```python
from build123d import *

# Parameters (mm, degrees)
F1_DEPTH = 3.175
F2_R     = 3.175
F3_DEPTH = 6.351


with BuildPart() as f1:
    # F0 (on Front) → F1 (new body, symmetric)
    with BuildSketch(Plane.XZ):
        with BuildLine():
            Line((0, 6.35), (-29.21, 6.35))
            ThreePointArc((-29.21, 6.35), (-33.700128, 4.490128), (-35.56, 0))
            ThreePointArc((-35.56, 0), (-33.700128, -4.490128), (-29.21, -6.35))
            Line((-29.21, -6.35), (0, -6.35))
            Line((0, -6.35), (29.21, -6.35))
            ThreePointArc((29.21, -6.35), (33.700128, -4.490128), (35.56, 0))
            ThreePointArc((35.56, 0), (33.700128, 4.490128), (29.21, 6.35))
            Line((29.21, 6.35), (0, 6.35))
        make_face()
    extrude(amount=F1_DEPTH, both=True)

    # F2 (on face) → F3 (cut, through all)
    with BuildSketch(Plane.XZ.offset(3.175)):
        with Locations((-29.21, 0)):
            Circle(F2_R)
        with Locations((29.21, 0)):
            Circle(F2_R)
    extrude(amount=-F3_DEPTH, mode=Mode.SUBTRACT)


solid = f1.part
```
Part model, mm, in its own coordinate system. Coordinates: 2 decimals unless noted, no trailing zeros. Loops run counter-clockwise (first coordinate to the right, second up) from the corner with the lowest first, then second, coordinate; pieces in that order, holes last. Notation, with made-up numbers: (23, 69.25) - (76, 69.25) arc R24 cw to (76, 86.25) - close; hole circle Ø3 at (35, 41.5). An arc over 180 degrees is marked (long way). Write item = value, one per line. Start each with the question number.
Item 1: Mould opens along Z. For faces 1 (the flat face through (0, 0, -6.35)), 2 (the flat face through (0, 0, 6.35)), 3 (the cylindrical face through (-32.38, -0.04, 0.14)) say: released by +Z, released by -Z, zero draft, split by the parting line, or undercut.
Item 2: Cut at C-C, the plane z = 2.5. Give the cut face in (x, y) (3 decimals), and give its area (3 significant figures).
Item 3: Cut at D-D, the plane z = 5.5. Give the cut face in (x, y) (3 decimals).
Item 4: Cut at B-B, the plane z = -0.75. Give the cut face in (x, y) (3 decimals), and give its area (3 significant figures).
Item 5: Cut at A-A, the plane y = 1.25. Give the cut face in (x, z) (3 decimals).
Item 6: Wall check: L1, parallel to Z at x = -29.21, y = 0.25 (3 decimals); L2, parallel to X at y = 2.25, z = -2.75. Give the ranges that are in metal, low to high. Write a range as from..to.
The answers:
q1.face_1 = released by -Z
q1.face_2 = released by +Z
q1.face_3 = undercut
q2.outline = (-35.047, -3.175) - (-31.167, -3.175) - (-31.167, 3.175) - (-35.047, 3.175) - close; (-27.253, -3.175) - (27.253, -3.175) - (27.253, 3.175) - (-27.253, 3.175) - close; (31.167, -3.175) - (35.047, -3.175) - (35.047, 3.175) - (31.167, 3.175) - close
q2.area = 395 mm2
q3.outline = (-32.384, -3.175) - (32.384, -3.175) - (32.384, 3.175) - (-32.384, 3.175) - close
q4.outline = (-35.516, -3.175) - (-32.295, -3.175) - (-32.295, 3.175) - (-35.516, 3.175) - close; (-26.125, -3.175) - (26.125, -3.175) - (26.125, 3.175) - (-26.125, 3.175) - close; (32.295, -3.175) - (35.516, -3.175) - (35.516, 3.175) - (32.295, 3.175) - close
q4.area = 373 mm2
q5.outline = (-29.21, -6.35) - (29.21, -6.35) arc R6.35 ccw to (29.21, 6.35) - (-29.21, 6.35) arc R6.35 ccw to start; hole circle Ø6.35 at (-29.21, 0); hole circle Ø6.35 at (29.21, 0)
q6.L1 = -6.35..-3.175, 3.175..6.35
q6.L2 = -34.93..-30.8, -27.62..27.62, 30.8..34.93
